```python
from build123d import *

# Parameters (mm, degrees)
BOSS_EXTRUDE1_DEPTH = 20
SKETCH2_R           = 2.5
CUT_EXTRUDE1_DEPTH  = 21
SKETCH3_R           = 2.5
CUT_EXTRUDE2_DEPTH  = 21
CUT_EXTRUDE3_START  = -2
SKETCH4_R           = 5
CUT_EXTRUDE3_DEPTH  = 19
CUT_EXTRUDE4_START  = -2
SKETCH5_R           = 5
CUT_EXTRUDE4_DEPTH  = 20


with BuildPart() as part:
    # Sketch1 → Boss-Extrude1 (new body)
    with BuildSketch(Plane(origin=(0, 0, 0), x_dir=(1, 0, 0), z_dir=(0, 1, 0))):
        Polygon((0, 0), (0, 20), (20, 0), align=None)
    extrude(amount=BOSS_EXTRUDE1_DEPTH)

    # Sketch2 → Cut-Extrude1 (cut, through all)
    with BuildSketch(Plane.XY):
        with Locations((10, 10)):
            Circle(SKETCH2_R)
    extrude(amount=-CUT_EXTRUDE1_DEPTH, mode=Mode.SUBTRACT)

    # Sketch3 → Cut-Extrude2 (cut, through all)
    with BuildSketch(Plane.ZY):
        with Locations((-10, 10)):
            Circle(SKETCH3_R)
    extrude(amount=-CUT_EXTRUDE2_DEPTH, mode=Mode.SUBTRACT)

    # Sketch4 → Cut-Extrude3 (cut, through all)
    with BuildSketch(Plane.ZY.offset(CUT_EXTRUDE3_START)):
        with Locations((-10, 10)):
            Circle(SKETCH4_R)
    extrude(amount=-CUT_EXTRUDE3_DEPTH, mode=Mode.SUBTRACT)

    # Sketch5 → Cut-Extrude4 (cut)
    with BuildSketch(Plane.XY.offset(CUT_EXTRUDE4_START)):
        with Locations((10, 10)):
            Circle(SKETCH5_R)
    extrude(amount=-CUT_EXTRUDE4_DEPTH, mode=Mode.SUBTRACT)


solid = part.part
```
For this review, take the finished solid that the model builds, in its own axes (mm). A direction names the side the tool comes from. Coordinates: 2 decimals unless noted, no trailing zeros. Loops run counter-clockwise (first coordinate to the right, second up) from the corner with the lowest first, then second, coordinate; pieces in that order, holes last.
1. Add section A-A, the plane y = 10. Give the boundary of the cut face in (x, z), then the cut area to 3 significant figures.
2. Mouldability with a two-part tool opening along X and no side actions: class faces 1 (the cylindrical face through (9.46, 7.56, -0.99)), 2 (the flat face through (8, 5, -12)), 3 (the cylindrical face through (0.99, 7.56, -10.54)) as +X half, -X half, draft (parallel to the pull), parting line (faces both ways), or undercut.
3. For faces 4 (the cylindrical face through (4.166, 8.085, -5.381)), 5 (the flat face through (0, 8, -12)), 6 (the flat face through (12, 8, -2)), list the 3-axis set-ups (+Z, -Z, +X, -X, +Y, -Y) from which the entire face can be reached by the end or side of a thin tool; tool diameter is ignored.
4. Add section B-B, the plane z = -3.5. Give the boundary of the cut face in (x, y).
5. For line 1 (Y direction, x = 0.6, z = -10); line 2 (Y direction, x = 5, z = -10); line 3 (Z direction, x = 11.25, y = 12.75), list the stretches that pass through material, from the lowest coordinate up.
6. Insertion check: P1, Ø1, axis at y = 8, z = -2.5, coming from the +X side; P2, Ø8, axis at x = 17.5, y = 17, coming from the -Z side; P3, Ø6, axis at y = 5, z = -7, coming from the +X side. Each pin has a flat end and moves straight along its axis. Give the tip position at first contact, or say it passes through.
7. Add section D-D, the plane y = 2.75. Give the boundary of the cut face in (x, z).
8. Add section C-C, the plane z = -14. Give the boundary of the cut face in (x, y), then the cut area to 3 significant figures.
Result:
1. outline: (0, -20) - (5, -15) - (2, -15) - (2, -12.5) - (0, -12.5) - close; (0, -7.5) - (2, -7.5) - (2, -5) - (5, -5) - (5, -2) - (7.5, -2) - (7.5, 0) - (0, 0) - close; (12.5, -2) - (15, -2) - (15, -5) - (20, 0) - (12.5, 0) - close
1. area: 70.0 mm2
2. face 1: undercut
2. face 2: +X half
2. face 3: draft
3. face 4: +X
3. face 5: +Z, -Z, -X, +Y, -Y
3. face 6: -Z
4. outline: (0, 0) - (16.5, 0) - (16.5, 20) - (0, 20) - close; hole circle Ø10 at (10, 10)
5. line 1: y = 0 to 7.5, 12.5 to 20
5. line 2: y = 0 to 5, 15 to 20
5. line 3: z = -2 to 0
6. P1: stops at x = 18
6. P2: stops at z = -6.5
6. P3: stops at x = 16
7. outline: (0, -20) - (20, 0) - (0, 0) - close
8. outline: (0, 0) - (6, 0) - (6, 7) - (2, 7) - (2, 13) - (6, 13) - (6, 20) - (0, 20) - close
8. area: 96.0 mm2
